Geometry check sheet. Reference: the model listing, model coordinates, mm. Coordinates: 2 decimals unless noted, no trailing zeros. Order: outer loops, then holes, each group sorted by start corner. A loop starts at its lowest first (then second) coordinate and runs counter-clockwise, first axis right, second up. Notation, with made-up numbers: (55.5, 50) - (75.5, 50) arc R17 ccw to (75.5, 74) - close; hole circle Ø5 at (66.25, 49). An arc over 180 degrees is marked (long way). Use CSV: the item, a comma, the result in double quotes. Start each with the question number.
1) Sectioned sample at B-B, the plane z = -23. Record the cut outline in (x, y).
2) Sectioned sample at A-A, the plane y = -11. Record the cut outline in (x, z), and give its area (3 significant figures).
3) Sectioned sample at D-D, the plane y = -20.5. Record the cut outline in (x, z).
4) Sectioned sample at C-C, the plane x = 17. Record the cut outline in (y, z), and give its area (3 significant figures).
5) Thickness scan on probe 1 along X at (y, z) = (-20, -29.25) (3 decimals); probe 2 along X at (y, z) = (-14.25, -27.25); probe 3 along Z at (x, y) = (-75, -22). Record the ranges inside material, lowest first. Write a range as [from, to].
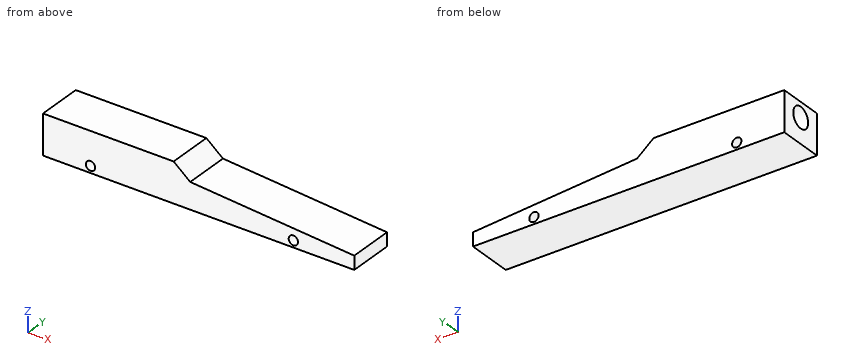
from build123d import *

# Parameters (mm, degrees)
F0_W      = 150
F0_H      = 20
F1_DEPTH  = 40
F2_R      = 5
F3_DEPTH  = 65
F4_W      = 150
F4_H      = 5
F5_DEPTH  = 20.001
F6_R      = 5
F7_DEPTH  = 55
F9_DEPTH  = 30.001
F10_W     = 4
F10_H     = 19.2120939866
F11_DEPTH = 150.001
F12_R     = 2.25
F13_DEPTH = 22.001


with BuildPart() as f1:
    # F0 (on Front) → F1 (new body)
    with BuildSketch(Plane.XZ):
        with Locations((-9.199729269, -22.2991868854)):
            Rectangle(F0_W, F0_H)
    extrude(amount=F1_DEPTH)

    # F2 (on face) → F3 (cut)
    with BuildSketch(Plane(origin=(-84.199729269, 0, 0), x_dir=(0, -1, 0), z_dir=(-1, 0, 0))):
        with Locations((20, 2.7008131146)):
            Circle(F2_R)
    extrude(amount=-F3_DEPTH, mode=Mode.SUBTRACT)

    # F4 (on face) → F5 (cut, through all)
    with BuildSketch(Plane.XY.offset(-12.2991868854)):
        with Locations((-9.199729269, -2.5)):
            Rectangle(F4_W, F4_H)
        with Locations((-9.199729269, -37.5)):
            Rectangle(F4_W, F4_H)
    extrude(amount=-F5_DEPTH, mode=Mode.SUBTRACT)

    # F6 (on face) → F7 (cut)
    with BuildSketch(Plane(origin=(-84.199729269, 0, 0), x_dir=(0, -1, 0), z_dir=(-1, 0, 0))):
        with Locations((20.0377495284, -20.2992462616)):
            Circle(F6_R)
    extrude(amount=-F7_DEPTH, mode=Mode.SUBTRACT)

    # F8 (on face) → F9 (cut, through all)
    with BuildSketch(Plane(origin=(0, -5, 0), x_dir=(-1, 0, 0), z_dir=(0, 1, 0))):
        Polygon((21.2375794259, -13.0870928988), (84.199729269, -13.0870928988), (84.199729269, -12.2991868854), (-65.800270731, -12.2991868854), (-65.800270731, -25.7824789733), (13.2570136338, -19.6707472205), align=None)
    extrude(amount=-F9_DEPTH, mode=Mode.SUBTRACT)

    # F10 (on face) → F11 (cut, through all)
    with BuildSketch(Plane(origin=(-84.199729269, 0, 0), x_dir=(0, -1, 0), z_dir=(-1, 0, 0))):
        with Locations((7, -22.6931398921)):
            Rectangle(F10_W, F10_H)
        with Locations((33, -22.6931398921)):
            Rectangle(F10_W, F10_H)
    extrude(amount=-F11_DEPTH, mode=Mode.SUBTRACT)

    # F12 (on face) → F13 (cut, through all)
    with BuildSketch(Plane(origin=(0, -9, 0), x_dir=(-1, 0, 0), z_dir=(0, 1, 0))):
        with Locations((-36.4439859986, -29.0491868854)):
            Circle(F12_R)
        with Locations((61.297416687, -29.0491868854)):
            Circle(F12_R)
    extrude(amount=-F13_DEPTH, mode=Mode.SUBTRACT)


solid = f1.part
Evaluation:
1,outline,"(-84.2, -31) - (29.81, -31) - (29.81, -9) - (-84.2, -9) - (-84.2, -15.83) - (-29.2, -15.83) - (-29.2, -24.25) - (-84.2, -24.25) - close"
2,outline,"(-84.2, -32.3) - (65.8, -32.3) - (65.8, -25.78) - (-13.26, -19.67) - (-21.24, -13.09) - (-84.2, -13.09) - close; hole circle Ø4.5 at (-61.3, -29.05); hole circle Ø4.5 at (36.44, -29.05)"
2,area,"2,060 mm²"
3,outline,"(-84.2, -32.3) - (65.8, -32.3) - (65.8, -25.78) - (-13.26, -19.67) - (-21.24, -13.09) - (-84.2, -13.09) - (-84.2, -15.32) - (-29.2, -15.32) - (-29.2, -25.28) - (-84.2, -25.28) - close; hole circle Ø4.5 at (-61.3, -29.05); hole circle Ø4.5 at (36.44, -29.05)"
4,outline,"(-31, -32.3) - (-9, -32.3) - (-9, -22.01) - (-31, -22.01) - close"
4,area,"226 mm²"
5,probe 1,"[-84.2, -63.538], [-59.056, 34.203], [38.685, 65.8]"
5,probe 2,"[-84.2, -62.65], [-59.95, 35.09], [37.8, 65.8]"
5,probe 3,"[-32.3, -24.9], [-15.7, -13.09]"
